Could you check a few things on this model? Use its own coordinates, in mm. A direction names the side the tool comes from. Give positions to 0.01 mm unless a question says otherwise; leave off trailing zeros. Order: outer loops, then holes, each group sorted by start corner. A loop starts at its lowest first (then second) coordinate and runs counter-clockwise, first axis right, second up.
(1) Imagine slicing it at B-B, the plane x = 5. Write out the boundary of the cut face in (y, z), then the cut area to 3 significant figures.
(2) On a 3-axis mill with a long thin cutter (end or side, diameter ignored), from which of +Z, -Z, +X, -X, +Y, -Y can I reach the whole of each face in a straight line? I mean faces 1 (the flat face through (5, 5.3, 1)), 2 (the cylindrical face through (16.03, -16.8, 4.09)). Say none if no direction works.
(3) Imagine slicing it at C-C, the plane y = -22.5. Write out the boundary of the cut face in (x, z).
(4) Imagine slicing it at D-D, the plane z = 5.75. State how many separate pieces and enclosed holes the cut face has, then the cut area to 3 significant figures.
(5) If I drill on probe 1 along Y at (x, z) = (0, 4.5); probe 2 along Y at (x, z) = (0, 0.4); probe 3 along Z at (x, y) = (-3, -11), over which ranges is the centre line in solid material (lowest first)?
(6) If we mould it in two halves opening along Y, with no side actions, what happens to faces 3 (the cylindrical face through (-22.89, -7.21, 4.09)), 4 (the flat face through (-13.99, 16.79, 4.6)), 5 (the flat face through (-1.7, -21.4, 8.3))? For each: released by +Y, released by -Y, zero draft, split by the parting line, or undercut.
(7) Will these pins go through, and if not, where does the flat tip stop? pin 1 (3 mm diameter, centred on x = 16, z = 5.5, fed in from +Y); pin 2 (4 mm diameter, centred on x = 19, z = 3.5, fed in from -Y); pin 3 (18 mm diameter, centred on x = 0, y = 0, fed in from +Z).
(8) Imagine slicing it at A-A, the plane y = 0. Write out the boundary of the cut face in (x, z), then the cut area to 3 significant figures.
from build123d import *

# Parameters (mm, degrees)
ESQUISSE1_R             = 24
ESQUISSE1_R_2           = 21
ESQUISSE1_R_3           = 0.9
BOSS_EXTRU_1_DEPTH      = 8.3
ESQUISSE2_R             = 21
BOSS_EXTRU_2_DEPTH      = 1
ENL_V_MAT_EXTRU_1_DEPTH = 35.941236383
ENL_V_MAT_EXTRU_2_DEPTH = 35.71728676


with BuildPart() as part:
    # Esquisse1 → Boss.-Extru.1 (new body)
    with BuildSketch(Plane.XY):
        with Locations(Location((0, 0, 0), (0, 0, 180))):
            Circle(ESQUISSE1_R)
        with Locations(Location((0, 0, 0), (0, 0, 180))):
            Circle(ESQUISSE1_R_2, mode=Mode.SUBTRACT)
        with Locations(Location((22.5, 0, 0), (0, 0, 180))):
            Circle(ESQUISSE1_R_3, mode=Mode.SUBTRACT)
        with Locations(Location((15.909902577, -15.909902577, 0), (0, 0, 180))):
            Circle(ESQUISSE1_R_3, mode=Mode.SUBTRACT)
        with Locations(Location((0, -22.5, 0), (0, 0, 180))):
            Circle(ESQUISSE1_R_3, mode=Mode.SUBTRACT)
        with Locations(Location((-15.909902577, -15.909902577, 0), (0, 0, 180))):
            Circle(ESQUISSE1_R_3, mode=Mode.SUBTRACT)
        with Locations(Location((-22.5, 0, 0), (0, 0, 180))):
            Circle(ESQUISSE1_R_3, mode=Mode.SUBTRACT)
        with Locations(Location((-15.909902577, 15.909902577, 0), (0, 0, 180))):
            Circle(ESQUISSE1_R_3, mode=Mode.SUBTRACT)
        with Locations(Location((0, 22.5, 0), (0, 0, 180))):
            Circle(ESQUISSE1_R_3, mode=Mode.SUBTRACT)
        with Locations(Location((15.909902577, 15.909902577, 0), (0, 0, 180))):
            Circle(ESQUISSE1_R_3, mode=Mode.SUBTRACT)
    extrude(amount=BOSS_EXTRU_1_DEPTH)

    # Esquisse2 → Boss.-Extru.2 (add)
    with BuildSketch(Plane.XY):
        with Locations(Location((0, 0, 0), (0, 0, 180))):
            Circle(ESQUISSE2_R)
    extrude(amount=BOSS_EXTRU_2_DEPTH)

    # Esquisse5 → Enlèv. mat.-Extru.1 (cut, through all)
    with BuildSketch(Plane(origin=(0, 0, 0), x_dir=(-1, 0, 0), z_dir=(0, 0, -1))):
        with BuildLine():
            ThreePointArc((-1.30820243, 6.85590272), (-2.670976724, -6.448308231), (5.772894113, 3.922816495))
            ThreePointArc((5.772894113, 3.922816495), (4.201710453, 10.143826361), (-1.30820243, 6.85590272))
        make_face()
    extrude(amount=-ENL_V_MAT_EXTRU_1_DEPTH, mode=Mode.SUBTRACT)

    # Esquisse6 → Enlèv. mat.-Extru.2 (cut, through all)
    with BuildSketch(Plane.XY.offset(1)):
        Polygon((-2.317366162, 22.579935361), (-14.327800085, 17.60505074), (-11.237259755, 10.143826361), (0.773174168, 15.118710982), align=None)
    extrude(amount=ENL_V_MAT_EXTRU_2_DEPTH, mode=Mode.SUBTRACT)


solid = part.part
Answer block:
1. outline: (-23.47, 0) - (-4.87, 0) - (-4.87, 1) - (-20.4, 1) - (-20.4, 8.3) - (-23.47, 8.3) - close; (4.87, 0) - (23.47, 0) - (23.47, 8.3) - (20.4, 8.3) - (20.4, 1) - (4.87, 1) - close
1. area: 82.1 mm2
2. face 1: +Z
2. face 2: +Z, -Z
3. outline: (-8.35, 0) - (-0.9, 0) - (-0.9, 8.3) - (-8.35, 8.3) - close; (0.9, 0) - (8.35, 0) - (8.35, 8.3) - (0.9, 8.3) - close
4. separate pieces: 1
4. enclosed holes: 9
4. area: 390 mm2
5. probe 1: y = -24 to -23.4, -21.6 to -21, 21 to 21.6, 23.4 to 24
5. probe 2: y = -24 to -23.4, -21.6 to -6.98, 9.43 to 21.6, 23.4 to 24
5. probe 3: z = 0 to 1
6. face 3: split by the parting line
6. face 4: undercut
6. face 5: zero draft
7. pin 1: stops at y = 19.12
7. pin 2: stops at y = -16.94
7. pin 3: stops at z = 1
8. outline: (-24, 0) - (-23.4, 0) - (-23.4, 8.3) - (-24, 8.3) - close; (-21.6, 0) - (-6.98, 0) - (-6.98, 1) - (-21, 1) - (-21, 8.3) - (-21.6, 8.3) - close; (6.98, 0) - (21.6, 0) - (21.6, 8.3) - (21, 8.3) - (21, 1) - (6.98, 1) - close; (23.4, 0) - (24, 0) - (24, 8.3) - (23.4, 8.3) - close
8. area: 48.0 mm2
